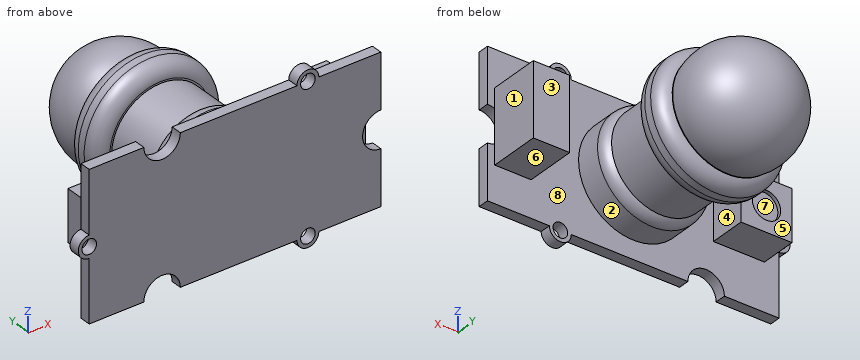
```python
from build123d import *

# Parameters (mm, degrees)
SKETCH1_W           = 40
SKETCH1_H           = 20
BOSS_EXTRUDE1_DEPTH = 1.5
SKETCH2_R           = 1.5
BOSS_EXTRUDE2_DEPTH = 1.5
SKETCH3_R           = 1
SKETCH3_R_2         = 2.5
CUT_EXTRUDE1_DEPTH  = 1.5
SKETCH4_W           = 7
SKETCH4_H           = 7
BOSS_EXTRUDE3_DEPTH = 5
SKETCH5_R           = 1.940753899
CUT_EXTRUDE2_DEPTH  = 0.5
SKETCH6_W           = 5
SKETCH6_H           = 10
BOSS_EXTRUDE4_DEPTH = 7
SKETCH7_R           = 7.5
BOSS_EXTRUDE5_DEPTH = 5
SKETCH8_R           = 6.75
BOSS_EXTRUDE6_DEPTH = 7
SKETCH9_R           = 9
BOSS_EXTRUDE7_DEPTH = 5
SKETCH11_R          = 7.5
BOSS_EXTRUDE8_DEPTH = 0.1
DOME1_FACE_RADIUS   = 7.5
DOME1_HEIGHT        = 10
FILLET2_R           = 2
FILLET4_R           = 2


with BuildPart() as part:
    # Sketch1 → Boss-Extrude1 (new body)
    with BuildSketch(Plane(origin=(0, 0, 0), x_dir=(1, 0, 0), z_dir=(0, 1, 0))):
        Rectangle(SKETCH1_W, SKETCH1_H)
    extrude(amount=BOSS_EXTRUDE1_DEPTH)

    # Sketch2 → Boss-Extrude2 (add)
    with BuildSketch(Plane(origin=(0, 1.5, 0), x_dir=(1, 0, 0), z_dir=(0, 1, 0))):
        with Locations((-20, 0)):
            Circle(SKETCH2_R)
        with Locations((10, 10)):
            Circle(SKETCH2_R)
        with Locations((10, -10)):
            Circle(SKETCH2_R)
    extrude(amount=-BOSS_EXTRUDE2_DEPTH)

    # Sketch3 → Cut-Extrude1 (cut)
    with BuildSketch(Plane(origin=(0, 1.5, 0), x_dir=(1, 0, 0), z_dir=(0, 1, 0))):
        with Locations(Location((-20, 0, 0), (0, 0, 270))):
            Circle(SKETCH3_R)
        with Locations(Location((10, -10, 0), (0, 0, 270))):
            Circle(SKETCH3_R)
        with Locations(Location((10, 10, 0), (0, 0, 270))):
            Circle(SKETCH3_R)
        with Locations((-10, -10)):
            Circle(SKETCH3_R_2)
        with Locations((-10, 10)):
            Circle(SKETCH3_R_2)
        with Locations((20, 0)):
            Circle(SKETCH3_R_2)
    extrude(amount=-CUT_EXTRUDE1_DEPTH, mode=Mode.SUBTRACT)

    # Sketch4 → Boss-Extrude3 (add)
    with BuildSketch(Plane(origin=(0, 1.5, 0), x_dir=(1, 0, 0), z_dir=(0, 1, 0))):
        with Locations((-14.5, 0)):
            Rectangle(SKETCH4_W, SKETCH4_H)
    extrude(amount=BOSS_EXTRUDE3_DEPTH)

    # Sketch5 → Cut-Extrude2 (cut)
    with BuildSketch(Plane(origin=(0, 6.5, 0), x_dir=(1, 0, 0), z_dir=(0, 1, 0))):
        with Locations(Location((-14.5, 0, 0), (0, 0, 270))):
            Circle(SKETCH5_R)
    extrude(amount=-CUT_EXTRUDE2_DEPTH, mode=Mode.SUBTRACT)

    # Sketch6 → Boss-Extrude4 (add)
    with BuildSketch(Plane(origin=(0, 1.5, 0), x_dir=(1, 0, 0), z_dir=(0, 1, 0))):
        with Locations((16.5, 0)):
            Rectangle(SKETCH6_W, SKETCH6_H)
    extrude(amount=BOSS_EXTRUDE4_DEPTH)

    # Sketch7 → Boss-Extrude5 (add)
    with BuildSketch(Plane(origin=(0, 1.5, 0), x_dir=(1, 0, 0), z_dir=(0, 1, 0))):
        with Locations(Location((0, 0, 0), (0, 0, 270))):
            Circle(SKETCH7_R)
    extrude(amount=BOSS_EXTRUDE5_DEPTH)

    # Sketch8 → Boss-Extrude6 (add)
    with BuildSketch(Plane(origin=(0, 6.5, 0), x_dir=(1, 0, 0), z_dir=(0, 1, 0))):
        with Locations(Location((0, 0, 0), (0, 0, 270))):
            Circle(SKETCH8_R)
    extrude(amount=BOSS_EXTRUDE6_DEPTH)

    # Sketch9 → Boss-Extrude7 (add)
    with BuildSketch(Plane(origin=(0, 13.5, 0), x_dir=(1, 0, 0), z_dir=(0, 1, 0))):
        with Locations(Location((0, 0, 0), (0, 0, 270))):
            Circle(SKETCH9_R)
    extrude(amount=BOSS_EXTRUDE7_DEPTH)

    # Sketch11 → Boss-Extrude8 (add)
    with BuildSketch(Plane(origin=(0, 18.5, 0), x_dir=(1, 0, 0), z_dir=(0, 1, 0))):
        with Locations(Location((0, 0, 0), (0, 0, 270))):
            Circle(SKETCH11_R)
    extrude(amount=BOSS_EXTRUDE8_DEPTH)

    # Dome1: a dome of height H over a round flat face of radius A is a cap of a sphere of radius (A * A + H * H) / (2 * H)
    dome1_r = (DOME1_FACE_RADIUS * DOME1_FACE_RADIUS + DOME1_HEIGHT * DOME1_HEIGHT) / (2 * DOME1_HEIGHT)
    dome1_base = Plane((0, 18.6, 0), z_dir=(0, 1, 0))
    with Locations(dome1_base.offset(DOME1_HEIGHT - dome1_r)):
        dome1_ball = Sphere(dome1_r, mode=Mode.PRIVATE)
    add(split(dome1_ball, bisect_by=dome1_base, keep=Keep.TOP, mode=Mode.PRIVATE))

    # Fillet2
    # the kernel refuses this fillet: 2 mm, written as the material it takes off along each edge
    with BuildSketch(Plane(origin=(0, 13.5, 0), x_dir=(0, 0, 1), z_dir=(-1, 0, 0))) as fillet2_piece_1:
        with BuildLine():
            CenterArc((9 - FILLET2_R, FILLET2_R), FILLET2_R, 270, 90)
            Line((9 - FILLET2_R, 0), (9 - FILLET2_R, -FILLET2_R * 0.02))
            Line((9 - FILLET2_R, -FILLET2_R * 0.02), (9 + FILLET2_R * 0.02, -FILLET2_R * 0.02))
            Line((9 + FILLET2_R * 0.02, -FILLET2_R * 0.02), (9 + FILLET2_R * 0.02, FILLET2_R))
            Line((9 + FILLET2_R * 0.02, FILLET2_R), (9, FILLET2_R))
        make_face()
    revolve(axis=Axis((0, 13.5, 0), (0, 1, 0)), mode=Mode.SUBTRACT)
    with BuildSketch(Plane(origin=(0, 18.5, 0), x_dir=(0, 0, 1), z_dir=(-1, 0, 0))) as fillet2_piece_2:
        with BuildLine():
            CenterArc((7, -1.936491673), FILLET2_R, 0, 75.522487814)
            Line((7.5, 0), (7.51, 0.038729833))
            ThreePointArc((7.51, 0.038729833), (8.25, 0.04), (9, 0.04))
            Line((9, 0.04), (9.04, 0))
            Line((9.04, 0), (9.04, -1.936491673))
            Line((9.04, -1.936491673), (9, -1.936491673))
        make_face()
    revolve(axis=Axis((0, 18.5, 0), (0, 1, 0)), mode=Mode.SUBTRACT)

    # Fillet4
    # the kernel refuses this fillet: 2 mm, written as the material it takes off along each edge
    with BuildSketch(Plane(origin=(0, 6.5, 0), x_dir=(0, 0, 1), z_dir=(-1, 0, 0))) as fillet4_piece_1:
        with BuildLine():
            CenterArc((5.5, -1.5612495), FILLET4_R, 0, 51.317812547)
            Line((7.5, -1.5612495), (7.54, -1.5612495))
            Line((7.54, -1.5612495), (7.54, 0))
            Line((7.54, 0), (7.5, 0.04))
            ThreePointArc((7.5, 0.04), (7.125, 0.04), (6.775, 0.03122499))
            Line((6.775, 0.03122499), (6.75, 0))
        make_face()
    revolve(axis=Axis((0, 6.5, 0), (0, 1, 0)), mode=Mode.SUBTRACT)


solid = part.part
```
Source: CAD feature listing. Evaluate the final solid. Frame: model axes, mm. Face numbers are marked on the shaded views. A direction names the side the tool comes from. Give positions to 0.01 mm unless a question says otherwise; leave off trailing zeros. Write each loop counter-clockwise with the first axis right and the second up, starting at its lowest first coordinate (ties: lowest second). Pieces come first, ordered by that corner, then holes.
1. Section query D-D (y = 11). Return the cut outline in (x, z), then the cut area to 3 significant figures.
2. Section query B-B (y = 8). Return the cut outline in (x, z).
3. Access query for the marked faces 4, 5, 6, 7 and 8. Directions: +Z, -Z, +X, -X, +Y, -Y. A direction counts if a zero-diameter tool reaches every point of the face in a straight line with its end or side. Return the directions, or none.
4. Material intervals for line 1 along X through (y, z) = (1.15, 0); line 2 along Y through (x, z) = (-15.5, 8.75); line 3 along Z through (x, y) = (-13.5, 3.25), sorted ascending.
5. Section query A-A (x = 10). Return the cut outline in (y, z).
6. First-contact query: pin 1 (1.5 mm diameter, centred on x = 11.5, z = 7.5, fed in from +Y); pin 2 (3 mm diameter, centred on y = 24.5, z = 7.5, fed in from +X); pin 3 (1.6 mm diameter, centred on x = -16.5, y = 0.5, fed in from -Z). Flat tips, straight axial feed; report the tip coordinate or a pass-through.
7. Pull-direction query (X, two-part tool) for the marked faces 1, 2 and 3; classes: +X half, -X half, draft (parallel to the pull), parting line (faces both ways), or undercut.
Output values:
1. outline: circle Ø13.5 at (0, 0)
1. area: 143 mm2
2. outline: circle Ø13.5 at (0, 0); (14, -5) - (19, -5) - (19, 5) - (14, 5) - close
3. face 4: +Z, -Z, +Y
3. face 5: +Z, -Z, -X, +Y
3. face 6: -Z, +X, +Y
3. face 7: +Y
3. face 8: none
4. line 1: x = -21.5 to -21, -19 to 17.5
4. line 2: y = 0 to 1.5
4. line 3: z = -3.5 to 3.5
5. outline: (0, -11.5) - (1.5, -11.5) - (1.5, -11) - (0, -11) - close; (0, -9) - (1.5, -9) - (1.5, 9) - (0, 9) - close; (0, 11) - (1.5, 11) - (1.5, 11.5) - (0, 11.5) - close
6. pin 1: stops at y = 1.5
6. pin 2: stops at x = 3.72
6. pin 3: stops at z = -10
7. face 1: +X half
7. face 2: undercut
7. face 3: draft
